Autodesk Inventor part; units mm, degrees
ref_plane "Plano de trabajo3" through (0, 0, -294.7) normal (0, 0, 1) x (1, 0, 0)
ref_plane "YZ Plane" through (0, 0, 0) normal (1, 0, 0) x (0, 1, 0)
ref_plane "XZ Plane" through (0, 0, 0) normal (0, 1, 0) x (-1, 0, 0)
sketch "Sketch1" plane through (0, 0, 0) normal (0, 0, 1) x (1, 0, 0)
  line L0 (-8.5, 42.6) -> (-6.1, 42.6)
  line L1 (-6.1, 36.1) -> (-8.5, 36.1)
  line L2 (-6.1, 36.1) -> (-6.1, 42.6)
  line L3 (-8.5, 37.35) -> (-8.5, 36.1)
  line L4 (-8.5, 41.35) -> (-8.5, 42.6)
  line L5 (-8.5, 37.35) -> (-9.2058, 37.35)
  line L6 (-8.5, 41.35) -> (-9.2058, 41.35)
  line L7 (-9.9, 42.36) -> (-9.2058, 41.35)
  line L8 (-9.9, 36.34) -> (-9.2058, 37.35)
  line L9 (-13.4, 36.34) -> (-9.9, 36.34)
  line L10 (-13.4, 36.34) -> (-13.4, 42.36)
  line L11 (-13.4, 42.36) -> (-9.9, 42.36)
  point P0 (-8.5, 41.975)
  point P1 (-6.1, 39.35)
  dimension "d27" = 6.5
  dimension "d28" = 2.4
  dimension "d29" = 2.4
  dimension "d35" = 111
  dimension "d36" = 4
  dimension "d37" = 6.02
  dimension "d38" = 0.7058
  dimension "d39" = 0.7058
  dimension "d43" = 3.01
  dimension "d44" = 2
  dimension "d63" = 3.5
  dimension "d64" = 3.5
extrude "Extrusion1" add sketch "Sketch1" against normal blind 589.4
ref_plane "Plano de trabajo3" through (0, 0, -294.7) normal (0, 0, 1) x (1, 0, 0)
sketch "Boceto2" plane through (-6.1, 36.1, 0) normal (1, 0, 0) x (0, 0, -1)
  line L0 (0, 0) -> (6.5, 6.5)
  line L1 (0, 6.5) -> (589.4, 6.5)
  line L2 (6.5, 6.5) -> (0, 6.5)
  line L3 (6.5, 6.5) -> (0, 6.5)
  line L4 (0, 0) -> (0, 6.5)
  line L5 (0, 0) -> (0, 6.5)
  point P0 (0, -36.1)
  dimension "d65" = 45
extrude "Extrusión3" cut sketch "Boceto2" against normal through all
mirror "Simetría3" about plane through (0, 0, -294.7) normal (0, 0, 1) of "Extrusión3"
properties part number "SP40-02 JUNTA INT 589 mm" material "Rubber"
Can you work these out from the model? Positions are in its coordinate system, mm. Give positions to 0.01 mm unless a question says otherwise; leave off trailing zeros. Write each loop counter-clockwise with the first axis right and the second up, starting at its lowest first coordinate (ties: lowest second). Pieces come first, ordered by that corner, then holes. Notation, with made-up numbers: (29, 4.5) -> (81, 4.5) arc R34 cw to (81, 35.5) -> close; hole circle Ø7 at (39.5, 65.25). An arc over 180 degrees is marked (long way). One line per item, written item: value.
Q1. Imagine slicing it at A-A on z = -367. Please give me the cut outline in (x, y).
Results found:
outline: (-13.4, 36.34) -> (-9.9, 36.34) -> (-9.21, 37.35) -> (-8.5, 37.35) -> (-8.5, 36.1) -> (-6.1, 36.1) -> (-6.1, 42.6) -> (-8.5, 42.6) -> (-8.5, 41.35) -> (-9.21, 41.35) -> (-9.9, 42.36) -> (-13.4, 42.36) -> close
Q2. Imagine slicing it at B-B on x = -12. Please give me the cut outline in (y, z).
Results found:
outline: (36.34, -589.16) -> (42.36, -583.14) -> (42.36, -6.26) -> (36.34, -0.24) -> close
Q3. For P1, Ø4, axis at x = -11.5, z = -336, coming from the -Y side; P2, Ø0.8, axis at x = -9, z = -400, coming from the -Y side; P3, Ø1, axis at x = -12, z = -333.5, coming from the +Y side, each with a flat end and sliding along its axis, tell me the tip position at first contact or that it passes through.
Results found:
P1: stops at y = 36.34
P2: stops at y = 37.07
P3: stops at y = 42.36
Q4. Please list where these lines run through material, in increasing order: line 1 (X direction, y = 37.25, z = -357); line 2 (X direction, y = 42.25, z = -205); line 3 (Y direction, x = -11.25, z = -358.5). Write a range as [from, to].
Results found:
line 1: x = [-13.4, -9.27], [-8.5, -6.1]
line 2: x = [-13.4, -9.82], [-8.5, -6.1]
line 3: y = [36.34, 42.36]
